Geometry check sheet. Reference: the model listing, model coordinates, mm. A direction names the side the tool comes from. Round coordinates to 2 decimals unless told otherwise and drop trailing zeros. Order: outer loops, then holes, each group sorted by start corner. A loop starts at its lowest first (then second) coordinate and runs counter-clockwise, first axis right, second up. Notation, with made-up numbers: (-19, -20.5) - (-6, -20.5) arc R13 cw to (-6, -10.5) - close; hole circle Ø3 at (28, 66.25). An arc over 180 degrees is marked (long way). Use a Markdown table: item, result. Add a question column.
(1) Access from +Z, -Z, +X, -X, +Y, -Y to the whole of each face (thin tool, end or side, straight path). Record for faces 1 (the face through (-3, 15, 0)), 2 (the face through (0, -25, 12.182)), 3 (the face through (-5.213, -12.465, 11.361)).
(2) Section check B-B on z = 0. Record the boundary of the cut face in (x, y).
(3) Mould release check, pull along Y, two halves, no side actions. Record for faces 4 (the face through (-6, -15, 9)), 5 (the face through (-8.63, -12.46, 7.24)), 6 (the face through (0, 30, -4)), 7 (the face through (0, -25, -10)): released by +Y, released by -Y, zero draft, split by the parting line, or undercut.
(4) Thickness scan on line 1 along X through (y, z) = (6, -0.25); line 2 along X through (y, z) = (-21.25, 0); line 3 along Z through (x, y) = (0, -28). Record the ranges inside material, lowest first. Write a range as [from, to].
(5) Gauge pin test, flat ends, axial feed: P1, Ø1.5, axis at y = 10, z = -3.5, coming from the -X side; P2, Ø1.5, axis at x = -1.5, z = 4, coming from the -Y side; P3, Ø6, axis at y = 7.5, z = 7.5, coming from the +X side. Record the tip position at first contact, or that the pin passes through.
(6) Section check C-C on x = -8.5. Record the boundary of the cut face in (y, z), then the cut area to 3 significant figures.
(7) Section check A-A on y = -32. Record the boundary of the cut face in (x, z), then the cut area to 3 significant figures.
(8) Section check D-D on x = 1.25. Record the boundary of the cut face in (y, z).
```python
from build123d import *

# Parameters (mm, degrees)
CUT_EXTRUDE2_DEPTH = 30
SKETCH6_W          = 2.5
SKETCH6_H          = 5
CUT_REVOLVE1_ANGLE = 50


with BuildPart() as part:
    # Sketch1 → Revolve1 (revolve)
    with BuildSketch(Plane.XY):
        Polygon((3, 30), (15, 30), (15, -40), (0, -40), (0, 0), (3, 0), align=None)
    revolve(axis=Axis((0, -40, 0), (0, 1, 0)))

    # Sketch3 → Cut-Extrude2 (cut)
    with BuildSketch(Plane.XZ.offset(40)):
        with BuildLine():
            Line((-2.5, 12.182458366), (-2.5, 9.682458366))
            ThreePointArc((-2.5, 9.682458366), (0, -10), (2.5, 9.682458366))
            Line((2.5, 9.682458366), (2.5, 12.182458366))
            Line((2.5, 12.182458366), (-2.5, 12.182458366))
        make_face()
    extrude(amount=-CUT_EXTRUDE2_DEPTH, mode=Mode.SUBTRACT)

    # Sketch6 → Cut-Revolve1 (revolve, cut)
    with BuildSketch(Plane(origin=(0, 0, 0), x_dir=(0, 0, -1), z_dir=(1, 0, 0))):
        with Locations((-11.25, -12.5)):
            Rectangle(SKETCH6_W, SKETCH6_H)
    revolve(axis=Axis((0, 0, 0), (0, -1, 0)), revolution_arc=CUT_REVOLVE1_ANGLE, mode=Mode.SUBTRACT)


solid = part.part
```
Check sheet entries:
| question | item | result |
|---|---|---|
| 1 | face 1 | +Y |
| 1 | face 2 | -Y |
| 1 | face 3 | none |
| 2 | outline | (-15, -40) - (-10, -40) - (-10, -10) - (10, -10) - (10, -40) - (15, -40) - (15, 30) - (3, 30) - (3, 0) - (-3, 0) - (-3, 30) - (-15, 30) - close |
| 3 | face 4 | undercut |
| 3 | face 5 | undercut |
| 3 | face 6 | released by +Y |
| 3 | face 7 | zero draft |
| 4 | line 1 | x = [-15, -2.99], [2.99, 15] |
| 4 | line 2 | x = [-15, -10], [10, 15] |
| 4 | line 3 | z = [-15, -10], [12.18, 15] |
| 5 | P1 | stops at x = -14.75 |
| 5 | P2 | stops at y = -10 |
| 5 | P3 | stops at x = 14.31 |
| 6 | outline | (-40, -12.36) - (30, -12.36) - (30, 12.36) - (-40, 12.36) - (-40, 5.27) - (-10, 5.27) - (-10, -5.27) - (-40, -5.27) - close; hole (-15, 7.13) - (-10, 7.13) - (-10, 9.17) - (-15, 9.17) - close |
| 6 | area | 1,400 mm2 |
| 7 | outline | circle Ø30 at (0, 0); hole (-2.5, 9.68) arc R10 ccw (long way) to (2.5, 9.68) - (2.5, 12.18) - (-2.5, 12.18) - close |
| 7 | area | 381 mm2 |
| 8 | outline | (-40, -14.95) - (30, -14.95) - (30, -2.73) - (0, -2.73) - (0, 2.73) - (30, 2.73) - (30, 14.95) - (-40, 14.95) - (-40, 12.18) - (-10, 12.18) - (-10, -9.92) - (-40, -9.92) - close |
